```python
from build123d import *

# Parameters (mm, degrees)
SKETCH1_R           = 1.524
SKETCH1_R_2         = 1.587500001
SKETCH1_R_3         = 1.5875
SKETCH1_R_4         = 1.523999993
SKETCH1_R_5         = 1.523999992
SKETCH1_R_6         = 1.587499996
SKETCH1_R_7         = 1.523999994
SKETCH1_R_8         = 1.587499994
SKETCH1_W           = 6.35
SKETCH1_H           = 3.175
SKETCH1_W_2         = 3.175
SKETCH1_H_2         = 6.35
BOSS_EXTRUDE1_DEPTH = 3.175


with BuildPart() as part:
    # Sketch1 → Boss-Extrude1 (new body)
    with BuildSketch(Plane(origin=(0, 0, 0), x_dir=(1, 0, 0), z_dir=(0, 1, 0))):
        with BuildLine():
            Line((-46.403884523, -61.196885763), (-49.15351518, -59.609385763))
            Line((-49.15351518, -59.609385763), (-47.56601518, -56.859755106))
            Line((-47.56601518, -56.859755106), (-50.315645837, -55.272255106))
            Line((-50.315645837, -55.272255106), (-51.903145837, -58.021885763))
            Line((-51.903145837, -58.021885763), (-57.402407151, -54.846885763))
            add(Edge.make_bspline(
                [(-63.499999964, -3.175000051), (-63.499999964, -15.74075082), (-71.94938611, -46.448183545), (-57.402407151, -54.846885763)],
                knots=[0, 0, 0, 0, 1, 1, 1, 1], degree=3))
            Line((-63.499999964, -3.175000051), (-63.499999964, -1.587500051))
            Line((-63.499999964, -1.587500051), (-60.324999964, -1.587500051))
            Line((-60.324999964, -1.587500051), (-60.324999964, 1.587499949))
            Line((-60.324999964, 1.587499949), (-63.499999964, 1.587499949))
            Line((-63.499999964, 1.587499949), (-63.499999964, 3.174999949))
            add(Edge.make_bspline(
                [(-23.44611538, 59.78686309), (-4.72729916, 27.364922338), (-63.499999964, 16.015994216), (-63.499999964, 3.174999949)],
                knots=[0, 0, 0, 0, 1, 1, 1, 1], degree=3))
            Line((-23.44611538, 59.78686309), (-29.79611538, 70.785385718))
            Line((-29.79611538, 70.785385718), (-27.046484723, 72.372885718))
            Line((-27.046484723, 72.372885718), (-25.458984723, 69.623255061))
            Line((-25.458984723, 69.623255061), (-22.709354066, 71.210755061))
            Line((-22.709354066, 71.210755061), (-24.296854066, 73.960385718))
            Line((-24.296854066, 73.960385718), (-18.797592752, 77.135385718))
            add(Edge.make_bspline(
                [(29.000369343, 56.58011314), (18.118109959, 62.862988525), (-4.250613793, 85.534087936), (-18.797592752, 77.135385718)],
                knots=[0, 0, 0, 0, 1, 1, 1, 1], degree=3))
            Line((29.000369343, 56.58011314), (30.375184671, 55.786363141))
            Line((30.375184671, 55.786363141), (28.787684671, 53.036732484))
            Line((28.787684671, 53.036732484), (31.537315328, 51.449232484))
            Line((31.537315328, 51.449232484), (33.124815328, 54.198863141))
            Line((33.124815328, 54.198863141), (34.499630657, 53.405113141))
            add(Edge.make_bspline(
                [(63.5, -9.5885), (26.062367559, -9.5885), (45.620257902, 46.984616007), (34.499630657, 53.405113141)],
                knots=[0, 0, 0, 0, 1, 1, 1, 1], degree=3))
            Line((63.5, -9.5885), (76.2, -9.5885))
            Line((76.2, -9.5885), (76.2, -12.7635))
            Line((76.2, -12.7635), (73.025, -12.7635))
            Line((73.025, -12.7635), (73.025, -15.9385))
            Line((73.025, -15.9385), (76.2, -15.9385))
            Line((76.2, -15.9385), (76.2, -22.2885))
            add(Edge.make_bspline(
                [(34.499630719, -53.405113134), (45.381890103, -47.122237749), (76.2, -39.085904436), (76.2, -22.2885)],
                knots=[0, 0, 0, 0, 1, 1, 1, 1], degree=3))
            Line((34.499630719, -53.405113134), (33.12481539, -54.198863134))
            Line((33.12481539, -54.198863134), (31.53731539, -51.449232477))
            Line((31.53731539, -51.449232477), (28.787684733, -53.036732477))
            Line((28.787684733, -53.036732477), (30.375184734, -55.786363134))
            Line((30.375184734, -55.786363134), (29.000369405, -56.580113134))
            add(Edge.make_bspline(
                [(-40.053884523, -50.198363135), (-21.335068302, -17.776422383), (17.87974216, -63.000610268), (29.000369405, -56.580113134)],
                knots=[0, 0, 0, 0, 1, 1, 1, 1], degree=3))
            Line((-40.053884523, -50.198363135), (-46.403884523, -61.196885763))
        make_face()
        with Locations((65.151, -14.351)):
            Circle(SKETCH1_R, mode=Mode.SUBTRACT)
        with Locations((49.403, -14.351)):
            Circle(SKETCH1_R, mode=Mode.SUBTRACT)
        with Locations((25.933399999, 44.917966413)):
            Circle(SKETCH1_R_2, mode=Mode.SUBTRACT)
        with Locations((20.9423, 36.273127627)):
            Circle(SKETCH1_R_3, mode=Mode.SUBTRACT)
        with Locations((-45.003830508, -49.246921076)):
            Circle(SKETCH1_R_4, mode=Mode.SUBTRACT)
        with Locations((-37.129830508, -35.608753018)):
            Circle(SKETCH1_R_5, mode=Mode.SUBTRACT)
        with Locations((25.933400062, -44.917966407)):
            Circle(SKETCH1_R_6, mode=Mode.SUBTRACT)
        with Locations((20.942300062, -36.273127622)):
            Circle(SKETCH1_R_3, mode=Mode.SUBTRACT)
        with Locations((-20.147169395, 63.597921031)):
            Circle(SKETCH1_R_7, mode=Mode.SUBTRACT)
        with Locations((-12.273169395, 49.959752973)):
            Circle(SKETCH1_R_4, mode=Mode.SUBTRACT)
        with Locations((-51.866799964, -5.1e-08)):
            Circle(SKETCH1_R_8, mode=Mode.SUBTRACT)
        with Locations((-41.884599964, -5.1e-08)):
            Circle(SKETCH1_R_3, mode=Mode.SUBTRACT)
        with Locations((57.277, -33.4645)):
            Circle(SKETCH1_R, mode=Mode.SUBTRACT)
        with Locations((-57.619607125, -32.871087053)):
            Circle(SKETCH1_R, mode=Mode.SUBTRACT)
        with Locations((0.342607125, 66.335587053)):
            Circle(SKETCH1_R, mode=Mode.SUBTRACT)
        Polygon((15.662315328, 23.952925913), (18.837315328, 29.452187227), (16.087684671, 31.039687227), (12.912684671, 25.540425913), align=None, mode=Mode.SUBTRACT)
        Polygon((-41.647895898, -40.259271724), (-43.235395898, -43.008902381), (-48.734657212, -39.833902381), (-47.147157212, -37.084271724), align=None, mode=Mode.SUBTRACT)
        with Locations((41.529, -14.351)):
            Rectangle(SKETCH1_W, SKETCH1_H, mode=Mode.SUBTRACT)
        Polygon((12.912684733, -25.540425908), (16.087684733, -31.039687222), (18.83731539, -29.452187222), (15.66231539, -23.952925908), align=None, mode=Mode.SUBTRACT)
        Polygon((-30.23051518, -26.833788331), (-33.40551518, -32.333049645), (-36.155145837, -30.745549645), (-32.980145837, -25.246288331), align=None, mode=Mode.SUBTRACT)
        with Locations((-31.749999964, -5e-08)):
            Rectangle(SKETCH1_W, SKETCH1_H, mode=Mode.SUBTRACT)
        Polygon((-8.123484723, 39.597288286), (-11.298484723, 45.0965496), (-8.548854066, 46.6840496), (-5.373854066, 41.184788286), align=None, mode=Mode.SUBTRACT)
        with Locations((57.277, -19.1135)):
            Rectangle(SKETCH1_W_2, SKETCH1_H_2, mode=Mode.SUBTRACT)
        Polygon((-14.041604102, 56.197771724), (-15.629104102, 58.947402381), (-10.129842788, 62.122402381), (-8.542342788, 59.372771724), align=None, mode=Mode.SUBTRACT)
    extrude(amount=BOSS_EXTRUDE1_DEPTH)


solid = part.part
```
Can you work these out from the model? Positions are in its coordinate system, mm. A direction names the side the tool comes from. Coordinates: 2 decimals unless noted, no trailing zeros.
Item 1: I'm going to push flat-ended pins straight in: pin 1 (3.5 mm diameter, centred on x = -45, z = 49.25, fed in from +Y) (3 decimals); pin 2 (0.8 mm diameter, centred on y = 1, z = -2.5, fed in from -X); pin 3 (1.6 mm diameter, centred on x = -31.5, y = 2, fed in from -Z); pin 4 (1 mm diameter, centred on x = 74.5, y = 1.5, fed in from -Z). Where does each tip first touch, or does it pass through?
Answers below:
pin 1: stops at y = 3.175
pin 2: stops at x = -63.5
pin 3: stops at z = -28.48
pin 4: stops at z = 9.59
Item 2: Please list where these lines run through material, in increasing order: L1, parallel to X at y = 1.3, z = 28; L2, parallel to Z at x = 24.5, y = 3; L3, parallel to Z at x = -31, y = 0.9 (1 decimal).
Answers below:
L1: x = -65.8 to -34.57, -30.9 to 14.33, 18 to 74.94
L2: z = -59.55 to -45.6, -44.24 to 44.24, 45.6 to 57.02
L3: z = -28.2 to -1.6, 1.6 to 26.4, 28.2 to 40.7
Item 3: Which directions (+Z, -Z, +X, -X, +Y, -Y) give clear straight access to the entire face, cutting with the end or side of a thin tool? Please do faces 4 (the face through (55.69, 2, 19)), 5 (the face through (75, 2, 15.938)), 6 (the face through (-62, 2, 1.588)).
Answers below:
face 4: +Y, -Y
face 5: +X, +Y, -Y
face 6: -X, +Y, -Y
Item 4: Suppose I cut it at A-A (y = 2.4). State how many separate pieces and enclosed holes the cut face has, then the cut area to 3 significant figures.
Answers below:
separate pieces: 1
enclosed holes: 24
area: 11,100 mm2
Item 5: If we mould it in two halves opening along Z, with no side actions, what happens to faces 1 (the face through (14.478, 1.565, 28.252)), 2 (the face through (-54.61, 1.57, 56.46)), 3 (the face through (-21.586, 1.565, -75.526))? For each: released by +Z, released by -Z, zero draft, split by the parting line, or undercut.
Answers below:
face 1: undercut
face 2: released by +Z
face 3: released by -Z
